Part model, mm, in its own coordinate system. Face numbers are marked on the shaded views. A direction names the side the tool comes from. Coordinates: 2 decimals unless noted, no trailing zeros. Loops run counter-clockwise (first coordinate to the right, second up) from the corner with the lowest first, then second, coordinate; pieces in that order, holes last.
```python
from build123d import *

# Parameters (mm, degrees)
SKETCH_1_W          = 20
SKETCH_1_H          = 27
EXTRUDE_1_DEPTH     = 3
SKETCH_2_W          = 2
SKETCH_2_H          = 27
EXTRUDE_2_DEPTH     = 34
SKETCH_3_W          = 2
SKETCH_3_H          = 27
EXTRUDE_3_DEPTH     = 34
SKETCH_4_W          = 3
SKETCH_4_H          = 2
EXTRUDE_4_DEPTH     = 34
SKETCH_6_W          = 7
SKETCH_6_H          = 27
EXTRUDE_5_DEPTH     = 2
SKETCH_7_R          = 1.7
CUT_EXTRUDE_1_DEPTH = 50.244289009
SKETCH_8_R          = 9.6
CUT_EXTRUDE_2_DEPTH = 50
CHAMFER_1_SIZE      = 4
FILLET_1_R          = 3


with BuildPart() as part:
    # 草图1 → 凸台-拉伸1 (new body)
    with BuildSketch(Plane(origin=(0, 0, 0), x_dir=(1, 0, 0), z_dir=(0, 1, 0))):
        with Locations((10, -13.5)):
            Rectangle(SKETCH_1_W, SKETCH_1_H)
    extrude(amount=EXTRUDE_1_DEPTH)

    # 草图2 → 凸台-拉伸2 (add)
    with BuildSketch(Plane(origin=(0, 3, 0), x_dir=(1, 0, 0), z_dir=(0, 1, 0))):
        with Locations((19, -13.5)):
            Rectangle(SKETCH_2_W, SKETCH_2_H)
    extrude(amount=EXTRUDE_2_DEPTH)

    # 草图3 → 凸台-拉伸3 (add)
    with BuildSketch(Plane(origin=(0, 3, 0), x_dir=(1, 0, 0), z_dir=(0, 1, 0))):
        with Locations((14, -13.5)):
            Rectangle(SKETCH_3_W, SKETCH_3_H)
    extrude(amount=EXTRUDE_3_DEPTH)

    # 草图4 → 凸台-拉伸4 (add)
    with BuildSketch(Plane(origin=(0, 3, 0), x_dir=(1, 0, 0), z_dir=(0, 1, 0))):
        with Locations((16.5, -1)):
            Rectangle(SKETCH_4_W, SKETCH_4_H)
        with Locations((16.5, -26)):
            Rectangle(SKETCH_4_W, SKETCH_4_H)
    extrude(amount=EXTRUDE_4_DEPTH)

    # 草图6 → 凸台-拉伸5 (add)
    with BuildSketch(Plane(origin=(0, 37, 0), x_dir=(1, 0, 0), z_dir=(0, 1, 0))):
        with Locations((16.5, -13.5)):
            Rectangle(SKETCH_6_W, SKETCH_6_H)
    extrude(amount=EXTRUDE_5_DEPTH)

    # 草图7 → 切除-拉伸1 (cut, through all)
    with BuildSketch(Plane(origin=(0, 3, 0), x_dir=(1, 0, 0), z_dir=(0, 1, 0))):
        with Locations(Location((5, -9, 0), (0, 0, 270))):
            Circle(SKETCH_7_R)
        with Locations(Location((5, -18, 0), (0, 0, 270))):
            Circle(SKETCH_7_R)
    extrude(amount=-CUT_EXTRUDE_1_DEPTH, mode=Mode.SUBTRACT)

    # 草图8 → 切除-拉伸2 (cut)
    with BuildSketch(Plane(origin=(20, 0, 0), x_dir=(0, 0, -1), z_dir=(1, 0, 0))):
        with Locations((-13.5, 22)):
            Circle(SKETCH_8_R)
    extrude(amount=-CUT_EXTRUDE_2_DEPTH, mode=Mode.SUBTRACT)

    # 倒角1
    chamfer_1_edges = [part.edges().sort_by_distance(p)[0] for p in [
        (13, 3, 13.5),
    ]]
    chamfer(chamfer_1_edges, length=CHAMFER_1_SIZE)

    # 圆角1
    fillet_1_edges = [part.edges().sort_by_distance(p)[0] for p in [
        (0, 1.5, 0),
        (0, 1.5, 27),
    ]]
    fillet(fillet_1_edges, radius=FILLET_1_R)


solid = part.part
```
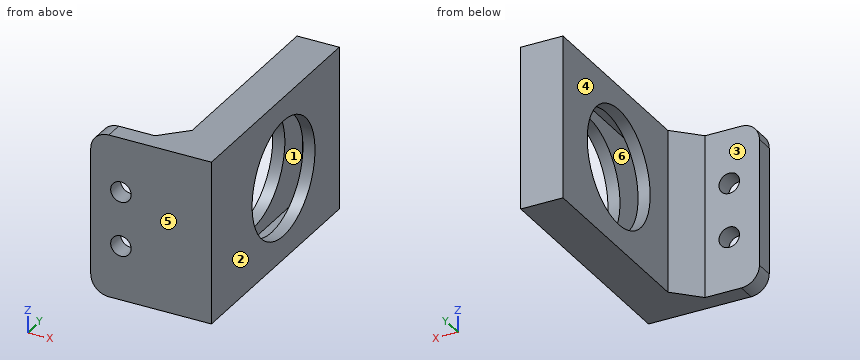
Q1. Saw through at B-B (x = 15.5). List the corners of the cut face in (y, z).
Q2. Saw through at D-D (y = 35). List the corners of the cut face in (x, z), plus the area to 3 significant figures.
Q3. Mould opens along X. For the marked faces 1, 2 and 3 say: released by +X, released by -X, zero draft, split by the parting line, or undercut.
Q4. Saw through at A-A (z = 13.5). List the corners of the cut face in (x, y), plus the area to 3 significant figures.
Q5. Probe line 1 (Y direction, x = 16.75, z = 18.5); line 2 (Y direction, x = 19.5, z = 13.5); line 3 (X direction, y = 9, z = 6.5). List the from-to ranges inside material, lowest first.
Q6. Saw through at C-C (y = 14.5). List the corners of the cut face in (x, z).
Q7. Drop flat-ended pins along their axis: P1, Ø7, axis at x = 2.5, z = 14.5, coming from the +Y side; P2, Ø12, axis at y = 16.5, z = 12.5, coming from the -X side. Give the stop position or say it passes through.
Q8. Tool access for the marked faces 4, 5 and 6: list every direction of +Z, -Z, +X, -X, +Y, -Y with a clear straight run to the whole face (end or side of a thin tool).
Checked values:
1. outline: (0, 0) - (39, 0) - (39, 27) - (0, 27) - close; hole (3, 2) - (37, 2) - (37, 25) - (3, 25) - close
2. outline: (13, 0) - (20, 0) - (20, 27) - (13, 27) - close; hole (15, 2) - (18, 2) - (18, 25) - (15, 25) - close
2. area: 120 mm2
3. face 1: undercut
3. face 2: released by +X
3. face 3: zero draft
4. outline: (0, 0) - (20, 0) - (20, 12.4) - (18, 12.4) - (18, 3) - (15, 3) - (15, 12.4) - (13, 12.4) - (13, 7) - (9, 3) - (0, 3) - close; (13, 31.6) - (15, 31.6) - (15, 37) - (18, 37) - (18, 31.6) - (20, 31.6) - (20, 39) - (13, 39) - close
4. area: 141 mm2
5. line 1: y = 0 to 3, 37 to 39
5. line 2: y = 0 to 12.4, 31.6 to 39
5. line 3: x = 13 to 15, 18 to 20
6. outline: (13, 0) - (20, 0) - (20, 7.51) - (18, 7.51) - (18, 2) - (15, 2) - (15, 7.51) - (13, 7.51) - close; (13, 19.49) - (15, 19.49) - (15, 25) - (18, 25) - (18, 19.49) - (20, 19.49) - (20, 27) - (13, 27) - close
7. P1: stops at y = 3
7. P2: stops at x = 13
8. face 4: +Z, -Z, -X, +Y
8. face 5: +Z, -Z, +X, -X, -Y
8. face 6: none
